```python
from build123d import *

# Parameters (mm, degrees)
SKETCH1_W                = 57.8
SKETCH1_H                = 24.4
BOSS_EXTRUDE1_DEPTH      = 2
SKETCH2_W                = 4
SKETCH2_H                = 24.4
BOSS_EXTRUDE2_DEPTH      = 24.4
SKETCH3_R                = 3
CUT_EXTRUDE1_DEPTH       = 78.293389523
SKETCH4_R                = 1.5
CUT_EXTRUDE2_DEPTH       = 91.459620286
SKETCH5_W                = 57.8
SKETCH5_H                = 24.4
BOSS_EXTRUDE3_DEPTH      = 2
SKETCH6_R                = 1.5
CUT_EXTRUDE3_DEPTH       = 13
SKETCH8_W                = 4
SKETCH8_H                = 24.4
BOSS_EXTRUDE4_DEPTH      = 25
BOSS_EXTRUDE5_DEPTH      = 25
SKETCH10_R               = 1.5
CUT_EXTRUDE4_DEPTH       = 91.623302203
SKETCH11_R               = 3.5
CUT_EXTRUDE5_DEPTH       = 78.500374605
BOSS_EXTRUDE6_DEPTH      = 61
BOSS_EXTRUDE6_DEPTH_BACK = 4
SKETCH14_W               = 4
SKETCH14_H               = 25


with BuildPart() as part:
    # Sketch1 → Boss-Extrude1 (new body)
    with BuildSketch(Plane.XY):
        with Locations((-43.243709624, -36.61462961)):
            Rectangle(SKETCH1_W, SKETCH1_H)
    extrude(amount=BOSS_EXTRUDE1_DEPTH)

    # Sketch2 → Boss-Extrude2 (add)
    with BuildSketch(Plane.XY.offset(2)):
        with Locations((-70.143709624, -36.61462961)):
            Rectangle(SKETCH2_W, SKETCH2_H)
    extrude(amount=BOSS_EXTRUDE2_DEPTH)

    # Sketch3 → Cut-Extrude1 (cut, through all)
    with BuildSketch(Plane(origin=(-68.143709624, 0, 0), x_dir=(0, 0, -1), z_dir=(1, 0, 0))):
        with Locations((-14.2, -36.61462961)):
            Circle(SKETCH3_R)
    extrude(amount=-CUT_EXTRUDE1_DEPTH, mode=Mode.SUBTRACT)

    # Sketch4 → Cut-Extrude2 (cut, through all)
    with BuildSketch(Plane.XY.offset(2)):
        with Locations((-60.143709624, -43.81462961)):
            Circle(SKETCH4_R)
        with Locations((-20.143709624, -43.81462961)):
            Circle(SKETCH4_R)
        with Locations((-20.143709624, -28.81462961)):
            Circle(SKETCH4_R)
        with Locations((-60.143709624, -28.81462961)):
            Circle(SKETCH4_R)
    extrude(amount=-CUT_EXTRUDE2_DEPTH, mode=Mode.SUBTRACT)

    # Sketch5 → Boss-Extrude3 (add)
    with BuildSketch(Plane(origin=(0, 0, 0), x_dir=(-1, 0, 0), z_dir=(0, 0, -1))):
        with Locations((43.243709624, -36.61462961)):
            Rectangle(SKETCH5_W, SKETCH5_H)
    extrude(amount=BOSS_EXTRUDE3_DEPTH)

    # Sketch6 → Cut-Extrude3 (cut)
    with BuildSketch(Plane.XY):
        with Locations((-60.143709624, -28.81462961)):
            Circle(SKETCH6_R)
        with Locations((-20.143709624, -28.81462961)):
            Circle(SKETCH6_R)
        with Locations((-20.143709624, -43.81462961)):
            Circle(SKETCH6_R)
        with Locations((-60.143709624, -43.81462961)):
            Circle(SKETCH6_R)
    extrude(amount=-CUT_EXTRUDE3_DEPTH, mode=Mode.SUBTRACT)

    # Sketch8 → Boss-Extrude4 (add)
    with BuildSketch(Plane.XY.offset(2)):
        with Locations((-70.143709624, -36.61462961)):
            Rectangle(SKETCH8_W, SKETCH8_H)
    extrude(amount=BOSS_EXTRUDE4_DEPTH)

    # Sketch9 → Boss-Extrude5 (add)
    with BuildSketch(Plane(origin=(0, -48.81462961, 0), x_dir=(-1, 0, 0), z_dir=(0, -1, 0))):
        Polygon((72.143709624, -27), (68.143709624, -27), (68.143709624, -2), (14.343709624, -2), (14.343709624, 2), (72.143709624, 2), align=None)
    extrude(amount=-BOSS_EXTRUDE5_DEPTH)

    # Sketch10 → Cut-Extrude4 (cut, through all)
    with BuildSketch(Plane.XY.offset(2)):
        with Locations((-58.143709624, -28.81462961)):
            Circle(SKETCH10_R)
        with Locations((-28.143709624, -28.81462961)):
            Circle(SKETCH10_R)
        with Locations((-28.143709624, -43.81462961)):
            Circle(SKETCH10_R)
        with Locations((-58.143709624, -43.81462961)):
            Circle(SKETCH10_R)
    extrude(amount=-CUT_EXTRUDE4_DEPTH, mode=Mode.SUBTRACT)

    # Sketch11 → Cut-Extrude5 (cut, through all)
    with BuildSketch(Plane(origin=(-68.143709624, 0, 0), x_dir=(0, 0, -1), z_dir=(1, 0, 0))):
        with Locations((-14.5, -36.31462961)):
            Circle(SKETCH11_R)
    extrude(amount=-CUT_EXTRUDE5_DEPTH, mode=Mode.SUBTRACT)

    # Sketch14 → Boss-Extrude6 (add, two sides: drawn at the far end of the back side and taken through both)
    with BuildSketch(Plane(origin=(-68.143709624, 0, 0), x_dir=(0, 0, -1), z_dir=(1, 0, 0)).offset(-BOSS_EXTRUDE6_DEPTH_BACK)):
        with Locations((0, -36.31462961)):
            Rectangle(SKETCH14_W, SKETCH14_H)
    extrude(amount=BOSS_EXTRUDE6_DEPTH + BOSS_EXTRUDE6_DEPTH_BACK)


solid = part.part
```
Design review of the part built by this model. Coordinates are the model's own, in mm. A direction names the side the tool comes from. Give positions to 0.01 mm unless a question says otherwise; leave off trailing zeros. Order: outer loops, then holes, each group sorted by start corner. A loop starts at its lowest first (then second) coordinate and runs counter-clockwise, first axis right, second up. Notation, with made-up numbers: (-20, 80) -> (3, 80) arc R25 cw to (3, 99) -> close; hole circle Ø6 at (-24.5, 11). An arc over 180 degrees is marked (long way). Write each question's results on one line, items separated by ' | '. Start each with the question number.
Q1. For pin 1 (6.5 mm diameter, centred on y = -36.31, z = 14.5, fed in from -X); pin 2 (2 mm diameter, centred on x = -22.5, y = -34.5, fed in from +Z); pin 3 (1.5 mm diameter, centred on y = -29.5, z = 17, fed in from +X), all flat-tipped, find the tip position at first contact; note any pin that passes through.
Q2. Add section B-B on y = -45.5. Give the boundary of the cut face in (x, z), and give its area (3 significant figures).
Q3. Add section C-C on x = -22.5. Give the boundary of the cut face in (y, z), and give its area (3 significant figures).
Q4. Mouldability with a two-part tool opening along Y and no side actions: class faces 3 (the cylindrical face through (-70.116, -32.844, 14.956)), 4 (the flat face through (-68.144, -33.7, 11.5)), 5 (the flat face through (-49.4, -23.815, 1.7)) as +Y half, -Y half, draft (parallel to the pull), parting line (faces both ways), or undercut.
Q5. Machinability: for faces 1 (the flat face through (-38, -36, 2)), 2 (the flat face through (-72.144, -39, 12)), which of the approach directions +Z, -Z, +X, -X, +Y, -Y give a long, thin tool a straight path to every point of the face, cutting with its end or side? Answer none if there is none.
Q6. Add section A-A on z = 14.5. Give the boundary of the cut face in (x, y), and give its area (3 significant figures).
Q7. Add section D-D on z = 4.25. Give the boundary of the cut face in (x, y), and give its area (3 significant figures).
Q8. Wall thickness on L1, parallel to Y at x = -70.3, z = 14.5; L2, parallel to Z at x = -51.5, y = -45.75; L3, parallel to X at y = -41.5, z = 10.25: over which ranges is each line inside the solid? List them lowest first. Write a range as from..to.
Found:
1) pin 1: passes through | pin 2: stops at z = 2 | pin 3: stops at x = -68.14
2) outline: (-72.14, -2) -> (-7.14, -2) -> (-7.14, 2) -> (-68.14, 2) -> (-68.14, 27) -> (-72.14, 27) -> close | area: 360 mm2
3) outline: (-48.81, -2) -> (-23.81, -2) -> (-23.81, 2) -> (-48.81, 2) -> close | area: 100 mm2
4) face 3: undercut | face 4: draft | face 5: +Y half
5) face 1: +Z, +X, +Y, -Y | face 2: +Z, -Z, -X, +Y, -Y
6) outline: (-72.14, -48.81) -> (-68.14, -48.81) -> (-68.14, -39.81) -> (-72.14, -39.81) -> close; (-72.14, -32.81) -> (-68.14, -32.81) -> (-68.14, -23.81) -> (-72.14, -23.81) -> close | area: 72.0 mm2
7) outline: (-72.14, -48.81) -> (-68.14, -48.81) -> (-68.14, -23.81) -> (-72.14, -23.81) -> close | area: 100 mm2
8) L1: y = -48.81..-39.81, -32.81..-23.81 | L2: z = -2..2 | L3: x = -72.14..-68.14
